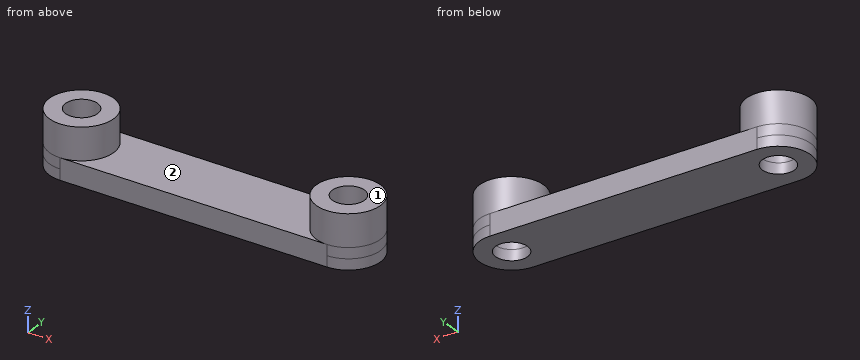
from build123d import *

# Parameters (mm, degrees)
SKETCH_1_R      = 1.5
EXTRUDE_1_DEPTH = 1
SKETCH_1_4_R    = 3
SKETCH_1_4_R_2  = 1.5
EXTRUDE_3_DEPTH = 4


with BuildPart() as part:
    # Sketch 1 → Extrude 1 (new, symmetric)
    with BuildSketch(Plane.XY):
        with BuildLine():
            Line((12.5, 3), (-12.5, 3))
            ThreePointArc((-12.5, 3), (-15.5, 0), (-12.5, -3))
            Line((-12.5, -3), (12.5, -3))
            ThreePointArc((12.5, -3), (15.5, 0), (12.5, 3))
        make_face()
        with Locations((-12.5, 0)):
            Circle(SKETCH_1_R, mode=Mode.SUBTRACT)
        with Locations((12.5, 0)):
            Circle(SKETCH_1_R, mode=Mode.SUBTRACT)
    extrude(amount=EXTRUDE_1_DEPTH, both=True)

    # Sketch 1_4 → Extrude 3 (add)
    # profile 1 of 2: a face of its own
    with BuildSketch(Plane.XY):
        with Locations(Location((12.5, 0, 0), (0, 0, 270))):
            Circle(SKETCH_1_4_R)
        with Locations((12.5, 0)):
            Circle(SKETCH_1_4_R_2, mode=Mode.SUBTRACT)
    # profile 2 of 2: a face of its own
    with BuildSketch(Plane.XY):
        with Locations(Location((-12.5, 0, 0), (0, 0, 90))):
            Circle(SKETCH_1_4_R)
        with Locations((-12.5, 0)):
            Circle(SKETCH_1_4_R_2, mode=Mode.SUBTRACT)
    extrude(amount=EXTRUDE_3_DEPTH)


solid = part.part
Work out the finished part from the listing and answer in its coordinate system (mm). Face numbers are marked on the shaded views. Round coordinates to 2 decimals unless told otherwise and drop trailing zeros. Write each loop counter-clockwise with the first axis right and the second up, starting at its lowest first coordinate (ties: lowest second). Pieces come first, ordered by that corner, then holes. Notation, with made-up numbers: M 31,63 L 77,63 A29 ccw 77,85 Z; hole C 63,66.25 d8. An arc over 180 degrees is marked long. Use a Markdown table: item, result.
1) Consider line 1 (X direction, y = 1.2, z = 2); line 2 (Y direction, x = 12.5, z = 1.9); line 3 (X direction, y = 0.65, z = 1.2). Determine where each line is inside the solid, lowest interval first. Write a range as [from, to].
Taken from the geometry:
| item | result |
|---|---|
| line 1 | x = [-15.25, -13.4], [-11.6, -9.75], [9.75, 11.6], [13.4, 15.25] |
| line 2 | y = [-3, -1.5], [1.5, 3] |
| line 3 | x = [-15.43, -13.85], [-11.15, -9.57], [9.57, 11.15], [13.85, 15.43] |
2) A flat-ended cylindrical pin translates along its axis: pin 1 (3 mm diameter, centred on x = -4, y = 1, fed in from +Z). Find the tip coordinate at first contact, or state that the pin passes through.
Taken from the geometry:
| item | result |
|---|---|
| pin 1 | stops at z = 1 |
3) The part is cut by section D-D on y = 1.9. Give the vertices of the cut face in (x, z).
Taken from the geometry:
| item | result |
|---|---|
| outline | M -14.82,-1 L 14.82,-1 L 14.82,4 L 10.18,4 L 10.18,1 L -10.18,1 L -10.18,4 L -14.82,4 Z |
4) The part is cut by section B-B on y = 0. Give the vertices of the cut face in (x, z).
Taken from the geometry:
| item | result |
|---|---|
| outline | M -15.5,-1 L -14,-1 L -14,4 L -15.5,4 Z; M -11,-1 L 11,-1 L 11,4 L 9.5,4 L 9.5,1 L -9.5,1 L -9.5,4 L -11,4 Z; M 14,-1 L 15.5,-1 L 15.5,4 L 14,4 Z |
5) Determine the mould class of the marked faces 1 and 2 for opening direction X: pulls with the +X half, pulls with the -X half, needs draft (parallel to the pull), parting line crosses it, or undercut.
Taken from the geometry:
| item | result |
|---|---|
| face 1 | needs draft |
| face 2 | undercut |
6) The part is cut by section C-C on x = -8. Give the vertices of the cut face in (y, z), plus the area to 3 significant figures.
Taken from the geometry:
| item | result |
|---|---|
| outline | M -3,-1 L 3,-1 L 3,1 L -3,1 Z |
| area | 12.0 mm2 |
7) The part is cut by section A-A on z = 0.4. Give the vertices of the cut face in (x, y).
Taken from the geometry:
| item | result |
|---|---|
| outline | M -12.5,-3 L 12.5,-3 A3 ccw 12.5,3 L -12.5,3 A3 ccw Z; hole C -12.5,0 d3; hole C 12.5,0 d3 |
